The model under review builds one solid part; all positions refer to its coordinate system, in mm. Coordinates: 2 decimals unless noted, no trailing zeros. Write each loop counter-clockwise with the first axis right and the second up, starting at its lowest first coordinate (ties: lowest second). Pieces come first, ordered by that corner, then holes. Notation, with made-up numbers: (68.25, 29) - (124.25, 29) arc R9 ccw to (124.25, 38) - close; hole circle Ø4 at (83, 30.25). An arc over 180 degrees is marked (long way). Return JSON: item names as keys, results as strings. Group by question number.
(1) To check wall thickness, follow L1, parallel to X at y = -5.75, z = 2; L2, parallel to Z at x = -1, y = -4; L3, parallel to Z at x = -66.5, y = -0.25. State the ranges of each line that lie inside material, in increasing order. Write a range as from..to.
(2) We need section D-D on x = -6. State the section outline as (y, z) points.
(3) For pin 1 Ø3 at (x, y) = (-56, -1.5) entering from +Z, flat-tipped, find the tip position at first contact; note if it passes through.
(4) We need section A-A on y = -4.25. State the section outline as (x, z) points, then the cut area to 3 significant figures.
(5) We need section B-B on x = -61. State the section outline as (y, z) points.
(6) Draft analysis for pull direction X (two halves, no side actions). For faces 1 (the face through (-70.174, -3.451, 0.479)), 2 (the face through (-30.06, -3.451, -30.214)), 3 (the face through (16, -7, 1)), state which applies: released by +X, released by -X, zero draft, split by the parting line, or undercut.
(7) We need section C-C on z = -2.5. State the section outline as (x, y) points, then the cut area to 3 significant figures.
```python
from build123d import *

# Parameters (mm, degrees)
F0_R     = 10.894565
F1_DEPTH = 7


with BuildPart() as f1:
    # F0 (on Front) → F1 (new body)
    with BuildSketch(Plane.XZ):
        with BuildLine():
            ThreePointArc((-43.45474, 0), (-48.092824, 11.197327), (-59.290151, 15.835411))
            ThreePointArc((-59.290151, 15.835411), (-75.125562, 0), (-59.290151, -15.835411))
            ThreePointArc((-59.290151, -15.835411), (-48.092824, -11.197327), (-43.45474, 0))
        make_face()
        with Locations((-59.290151, 0)):
            Circle(F0_R, mode=Mode.SUBTRACT)
        Polygon((59.290151, -15.835411), (0, -15.835411), (-59.290151, -15.835411), (0, -45), align=None)
        Polygon((-59.290151, 15.835411), (0, 15.835411), (59.290151, 15.835411), (0, 45), align=None)
        with BuildLine():
            ThreePointArc((0, 15.835411), (11.197327, 11.197327), (15.835411, 0))
            ThreePointArc((15.835411, 0), (11.197327, -11.197327), (0, -15.835411))
            Line((0, -15.835411), (59.290151, -15.835411))
            ThreePointArc((59.290151, -15.835411), (43.45474, 0), (59.290151, 15.835411))
            Line((59.290151, 15.835411), (0, 15.835411))
        make_face()
        with BuildLine():
            ThreePointArc((0, -15.835411), (-15.835411, 0), (0, 15.835411))
            Line((0, 15.835411), (-59.290151, 15.835411))
            ThreePointArc((-59.290151, 15.835411), (-48.092824, 11.197327), (-43.45474, 0))
            ThreePointArc((-43.45474, 0), (-48.092824, -11.197327), (-59.290151, -15.835411))
            Line((-59.290151, -15.835411), (0, -15.835411))
        make_face()
        with BuildLine():
            ThreePointArc((75.125562, 0), (70.487478, 11.197327), (59.290151, 15.835411))
            ThreePointArc((59.290151, 15.835411), (43.45474, 0), (59.290151, -15.835411))
            ThreePointArc((59.290151, -15.835411), (70.487478, -11.197327), (75.125562, 0))
        make_face()
        with Locations((59.290151, 0)):
            Circle(F0_R, mode=Mode.SUBTRACT)
        with BuildLine():
            ThreePointArc((0, -15.835411), (11.197327, -11.197327), (15.835411, 0))
            ThreePointArc((15.835411, 0), (11.197327, 11.197327), (0, 15.835411))
            ThreePointArc((0, 15.835411), (-15.835411, 0), (0, -15.835411))
        make_face()
        Circle(F0_R, mode=Mode.SUBTRACT)
    extrude(amount=F1_DEPTH)


solid = f1.part
```
Ans:
{
 "1": {"L1": "-75..-70, -48.58..-10.71, 10.71..48.58, 70..75", "L2": "-44.51..-10.85, 10.85..44.51", "L3": "-14.1..-8.17, 8.17..14.1"},
 "2": {"outline": "(-7, -42.05) - (0, -42.05) - (0, -9.09) - (-7, -9.09) - close; (-7, 9.09) - (0, 9.09) - (0, 42.05) - (-7, 42.05) - close"},
 "3": {"pin 1": "z = 18.19"},
 "4": {"outline": "(-59.29, -15.84) - (0, -45) - (59.29, -15.84) arc R15.84 ccw to (75.13, 0) arc R15.84 ccw to (59.29, 15.84) - (0, 45) - (-59.29, 15.84) arc R15.84 ccw to start; hole circle Ø21.79 at (-59.29, 0); hole circle Ø21.79 at (0, 0); hole circle Ø21.79 at (59.29, 0)", "area": "6,880 mm²"},
 "5": {"outline": "(-7, -15.74) - (0, -15.74) - (0, -10.76) - (-7, -10.76) - close; (-7, 10.76) - (0, 10.76) - (0, 15.74) - (-7, 15.74) - close"},
 "6": {"face 1": "undercut", "face 2": "released by -X", "face 3": "zero draft"},
 "7": {"outline": "(-74.93, -7) - (-69.89, -7) - (-69.89, 0) - (-74.93, 0) - close; (-48.69, -7) - (-10.6, -7) - (-10.6, 0) - (-48.69, 0) - close; (10.6, -7) - (48.69, -7) - (48.69, 0) - (10.6, 0) - close; (69.89, -7) - (74.93, -7) - (74.93, 0) - (69.89, 0) - close", "area": "604 mm²"}
}
